Geometry: final body of the model. Coordinates: model frame, mm. A direction names the side the tool comes from. Give positions to 0.01 mm unless a question says otherwise; leave off trailing zeros. Write each loop counter-clockwise with the first axis right and the second up, starting at its lowest first coordinate (ties: lowest second). Pieces come first, ordered by that corner, then holes. Notation, with made-up numbers: M -20,88.25 L -12,88.25 A10 ccw -12,95.25 Z; hole C 20,-9 d1. An arc over 180 degrees is marked long. Use a Markdown table: item, result. Add a question column.
(1) Draft query along X for faces 4 (the flat face through (25.311, -85.636, 3.131)), 5 (the flat face through (0, -50, 0)), 6 (the flat face through (-6.35, -32, 3)), 7 (the flat face through (-25.311, -85.636, 3.131)). Return one class per face: released by +X, released by -X, zero draft, split by the parting line, or undercut.
(2) Pin query (flat end, axial travel): pin 1 Ø3 at (y, z) = (-32.5, 4.5) entering from -X; pin 2 Ø1.9 at (x, z) = (1.5, 3) entering from -Y. Return the tip coordinate at first contact, or that it passes through.
(3) Material intervals for L1, parallel to X at y = -92, z = 0.5 (3 decimals); L2, parallel to X at y = -27, z = 2; L3, parallel to X at y = -81, z = 5.75 (3 decimals), sorted ascending.
(4) Cut plane B-B (z = 2.5). Output: boundary loops of the cut face in (x, y) (3 decimals).
(5) Reachability of faces 1 (the flat face through (0, -50, 6.35)), 2 (the flat face through (6.35, -32, 3)), 3 (the flat face through (0, -63.5, 3)) from +Z, -Z, +X, -X, +Y, -Y: full face, straight path, thin tool, end or side. Return the list, or none.
(6) Cut plane A-A (y = -74.5). Output: boundary loops of the cut face in (x, z) (3 decimals), plus the area to 3 significant figures.
(7) Cut plane C-C (y = -44). Output: boundary loops of the cut face in (x, z).
(8) Cut plane D-D (x = 11). Output: boundary loops of the cut face in (y, z) (3 decimals).
```python
from build123d import *

# Parameters (mm, degrees)
F0_W     = 6.35
F0_H     = 63.5
F1_DEPTH = 6.35
F3_DEPTH = 6.35


# Not quite as in the source:
# - a feature names something its author has since deleted; it is built from what else it names


with BuildPart() as f1:
    # F0 (on Top) → F1 (new body)
    with BuildSketch(Plane.XY):
        with Locations((-3.175, -31.75)):
            Rectangle(F0_W, F0_H)
    extrude(amount=F1_DEPTH)

    # F2 (on face) → F3 (join)
    with BuildSketch(Plane(origin=(0, 0, 0), x_dir=(1, 0, 0), z_dir=(0, 0, -1))):
        Polygon((-4.9710512242, 61.7039487758), (-3.175, 63.5), (-48.0762806053, 108.4012806053), (-49.8723318296, 106.6052293811), align=None)
    extrude(amount=-F3_DEPTH)

    # F4: F1 across plane


with BuildPart() as f1_1:
    add(f1.part)
    add(f1.part.mirror(Plane.YZ))


solid = f1_1.part
```
Answer list:
| question | item | result |
|---|---|---|
| 1 | face 4 | undercut |
| 1 | face 5 | zero draft |
| 1 | face 6 | released by -X |
| 1 | face 7 | undercut |
| 2 | pin 1 | x = -6.35 |
| 2 | pin 2 | y = -63.5 |
| 3 | L1 | -35.267 to -31.675, 31.675 to 35.267 |
| 3 | L2 | -6.35 to 6.35 |
| 3 | L3 | -24.267 to -20.675, 20.675 to 24.267 |
| 4 | outline | M -49.872,-106.605 L -48.076,-108.401 L -3.175,-63.5 L 3.175,-63.5 L 48.076,-108.401 L 49.872,-106.605 L 6.35,-63.083 L 6.35,0 L -6.35,0 L -6.35,-63.083 Z |
| 5 | face 1 | +Z, +X, -X, +Y, -Y |
| 5 | face 2 | +Z, -Z, +X, +Y |
| 5 | face 3 | +Z, -Z, -Y |
| 6 | outline | M -17.767,0 L -14.175,0 L -14.175,6.35 L -17.767,6.35 Z; M 14.175,0 L 17.767,0 L 17.767,6.35 L 14.175,6.35 Z |
| 6 | area | 45.6 mm² |
| 7 | outline | M -6.35,0 L 6.35,0 L 6.35,6.35 L -6.35,6.35 Z |
| 8 | outline | M -71.325,0 L -67.733,0 L -67.733,6.35 L -71.325,6.35 Z |
